Can you work these out from the drawing? Everything is in mm from the part's minimum corner. A direction names the side the tool comes from. Round coordinates to 2 decimals unless told otherwise and drop trailing zeros. Order: outer loops, then holes, each group sorted by start corner. A loop starts at its lowest first (then second) coordinate and runs counter-clockwise, first axis right, second up. Notation, with made-up numbers: (-12, 33) -> (17, 33) arc R21 cw to (17, 50) -> close; hole circle Ø7 at (-23.75, 72.25). An arc over 180 degrees is marked (long way). One line per item, written item: value.
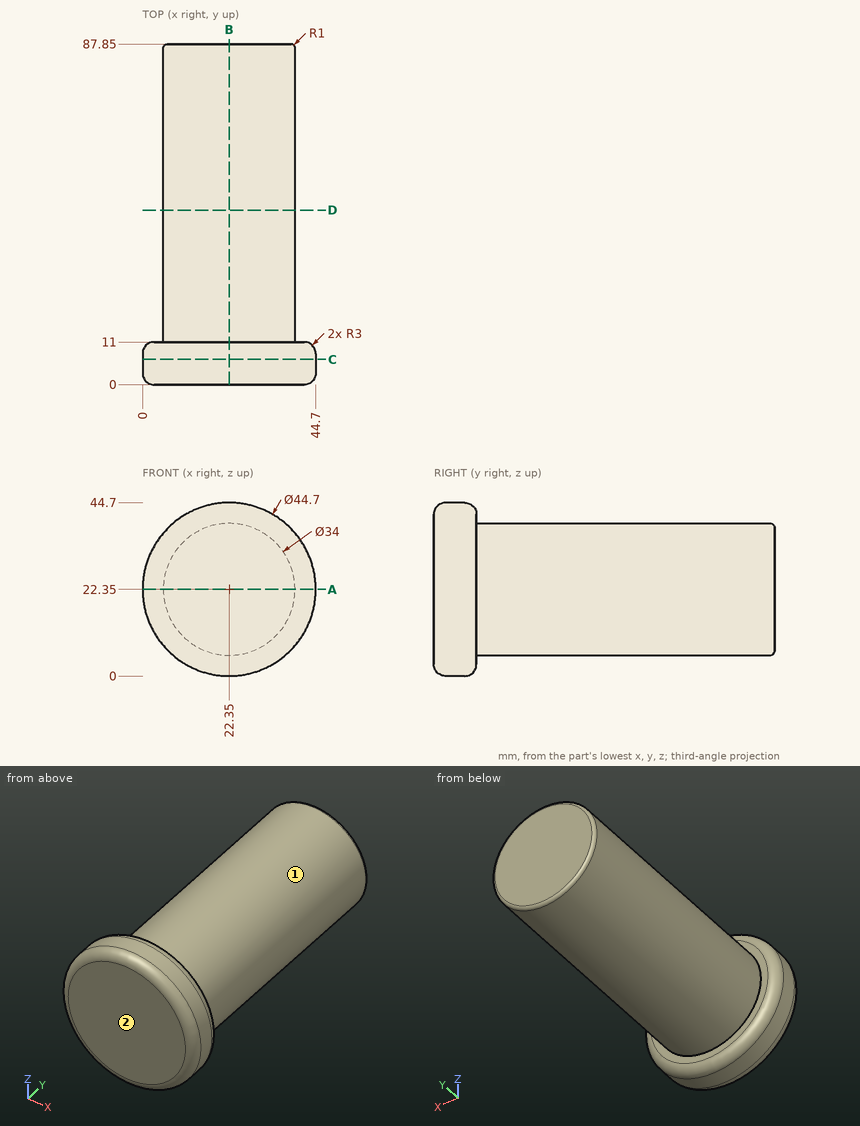
Q1. I want a section at D-D on y = 45. List the corners of the cut face in (x, z) for me.
Answers below:
outline: circle Ø34 at (22.35, 22.35)
Q2. On a 3-axis mill with a long thin cutter (end or side, diameter ignored), from which of +Z, -Z, +X, -X, +Y, -Y can I reach the whole of each face in a straight line? I mean the marked faces 1 and 2. Say none if no direction works.
Answers below:
face 1: +Y
face 2: +Z, -Z, +X, -X, -Y
Q3. I want a section at A-A on z = 22.35. List the corners of the cut face in (x, y) for me, plus the area to 3 significant figures.
Answers below:
outline: (0, 3) arc R3 ccw to (3, 0) -> (41.7, 0) arc R3 ccw to (44.7, 3) -> (44.7, 8) arc R3 ccw to (41.7, 11) -> (39.35, 11) -> (39.35, 86.85) arc R1 ccw to (38.35, 87.85) -> (6.35, 87.85) arc R1 ccw to (5.35, 86.85) -> (5.35, 11) -> (3, 11) arc R3 ccw to (0, 8) -> close
area: 3,100 mm^2
Q4. I want a section at B-B on x = 22.35. List the corners of the cut face in (y, z) for me.
Answers below:
outline: (0, 3) arc R3 ccw to (3, 0) -> (8, 0) arc R3 ccw to (11, 3) -> (11, 5.35) -> (86.85, 5.35) arc R1 ccw to (87.85, 6.35) -> (87.85, 38.35) arc R1 ccw to (86.85, 39.35) -> (11, 39.35) -> (11, 41.7) arc R3 ccw to (8, 44.7) -> (3, 44.7) arc R3 ccw to (0, 41.7) -> close
Q5. Will these pins go through, and if not, where does the flat tip stop? pin 1 Ø8 at (y, z) = (10.5, 15.5) entering from +X; pin 2 Ø2 at (x, y) = (18, 50.5) entering from -Z; pin 3 Ø12 at (y, z) = (19.5, 16) entering from +X.
Answers below:
pin 1: x = 44.41
pin 2: z = 5.68
pin 3: x = 39.35
Q6. I want a section at C-C on y = 6.5. List the corners of the cut face in (x, z) for me.
Answers below:
outline: circle Ø44.7 at (22.35, 22.35)
Q7. Please list where these lines run through material, in increasing order: line 1 along Y through (x, z) = (22, 4); line 2 along X through (y, z) = (77, 29.5); line 3 along Z through (x, y) = (22, 33).
Answers below:
line 1: 0 to 11
line 2: 6.93 to 37.77
line 3: 5.35 to 39.35
